Read the model definition and answer for the solid it produces. Units are mm, in the model's axes. Coordinates: 2 decimals unless noted, no trailing zeros. Loops run counter-clockwise (first coordinate to the right, second up) from the corner with the lowest first, then second, coordinate; pieces in that order, holes last.
from build123d import *

# Parameters (mm, degrees)
SKETCH1_R           = 4
SKETCH1_R_2         = 1.5
BOSS_EXTRUDE1_DEPTH = 2


with BuildPart() as part:
    # Sketch1 → Boss-Extrude1 (new body)
    with BuildSketch(Plane(origin=(0, 0, 0), x_dir=(1, 0, 0), z_dir=(0, 1, 0))):
        with BuildLine():
            Line((19, -12.5), (-19, -12.5))
            ThreePointArc((-19, -12.5), (-31.5, 0), (-19, 12.5))
            Line((-19, 12.5), (19, 12.5))
            ThreePointArc((19, 12.5), (31.5, 0), (19, -12.5))
        make_face()
        with Locations((-19, 0)):
            Circle(SKETCH1_R, mode=Mode.SUBTRACT)
        with Locations((19, 0)):
            Circle(SKETCH1_R, mode=Mode.SUBTRACT)
        with Locations((-19, 7)):
            Circle(SKETCH1_R_2, mode=Mode.SUBTRACT)
        with Locations((-12, 0)):
            Circle(SKETCH1_R_2, mode=Mode.SUBTRACT)
        with Locations((-26, 0)):
            Circle(SKETCH1_R_2, mode=Mode.SUBTRACT)
        with Locations((-19, -7)):
            Circle(SKETCH1_R_2, mode=Mode.SUBTRACT)
        with Locations((12, 0)):
            Circle(SKETCH1_R_2, mode=Mode.SUBTRACT)
        with Locations((19, 7)):
            Circle(SKETCH1_R_2, mode=Mode.SUBTRACT)
        with Locations((26, 0)):
            Circle(SKETCH1_R_2, mode=Mode.SUBTRACT)
        with Locations((19, -7)):
            Circle(SKETCH1_R_2, mode=Mode.SUBTRACT)
    extrude(amount=BOSS_EXTRUDE1_DEPTH)


solid = part.part
Q1. A cutting plane is placed at B-B (x = -12). Give the vertices of the cut face in (y, z), then the cut area to 3 significant figures.
Findings below:
outline: (0, -12.5) - (2, -12.5) - (2, -1.5) - (0, -1.5) - close; (0, 1.5) - (2, 1.5) - (2, 12.5) - (0, 12.5) - close
area: 44.0 mm2
Q2. Straight lines are drawn through the part: probe 1 along Z at (x, y) = (-19, 1.5); probe 2 along X at (y, z) = (0.6, 7); probe 3 along X at (y, z) = (0.5, -3.25). For each, find the intervals that lie inside material, in ascending order.
Findings below:
probe 1: z = -12.5 to -8.5, -5.5 to -4, 4 to 5.5, 8.5 to 12.5
probe 2: x = -29.36 to -20.5, -17.5 to 17.5, 20.5 to 29.36
probe 3: x = -31.07 to -21.33, -16.67 to 16.67, 21.33 to 31.07
Q3. A cutting plane is placed at C-C (y = 1.55). Count the separate pieces of the cut face and the enclosed holes in it, then the cut area to 3 significant figures.
Findings below:
separate pieces: 1
enclosed holes: 10
area: 1,280 mm2
Q4. A cutting plane is placed at D-D (z = 7). Give the vertices of the cut face in (x, y).
Findings below:
outline: (-29.36, 0) - (-20.5, 0) - (-20.5, 2) - (-29.36, 2) - close; (-17.5, 0) - (17.5, 0) - (17.5, 2) - (-17.5, 2) - close; (20.5, 0) - (29.36, 0) - (29.36, 2) - (20.5, 2) - close
Q5. A cutting plane is placed at A-A (z = 0). Give the vertices of the cut face in (x, y).
Findings below:
outline: (-31.5, 0) - (-27.5, 0) - (-27.5, 2) - (-31.5, 2) - close; (-24.5, 0) - (-23, 0) - (-23, 2) - (-24.5, 2) - close; (-15, 0) - (-13.5, 0) - (-13.5, 2) - (-15, 2) - close; (-10.5, 0) - (10.5, 0) - (10.5, 2) - (-10.5, 2) - close; (13.5, 0) - (15, 0) - (15, 2) - (13.5, 2) - close; (23, 0) - (24.5, 0) - (24.5, 2) - (23, 2) - close; (27.5, 0) - (31.5, 0) - (31.5, 2) - (27.5, 2) - close
Q6. Determine the mould class of faces 1 (the face through (-13.5, 0.99, -0.07)), 2 (the face through (-31.497, 0.986, 0.275)), 3 (the face through (0, 2, 0)) for opening direction X: +X half, -X half, draft (parallel to the pull), parting line (faces both ways), or undercut.
Findings below:
face 1: undercut
face 2: -X half
face 3: draft
